Autodesk Inventor part; units mm, degrees
ref_plane "YZ Plane" through (0, 0, 0) normal (1, 0, 0) x (0, 1, 0)
ref_plane "XZ Plane" through (0, 0, 0) normal (0, 1, 0) x (-1, 0, 0)
ref_plane "XY Plane" through (0, 0, 0) normal (0, 0, 1) x (1, 0, 0)
sketch "Esboço1" plane through (0, 0, 0) normal (0, 1, 0) x (-1, 0, 0)
  line L0 (-29, 17) -> (29, 17)
  line L1 (29, 17) -> (29, -17)
  line L2 (29, -17) -> (-29, -17)
  line L3 (-29, -17) -> (-29, 17)
  line L4 (-29, 17) -> (29, -17) construction
  line L5 (29, 17) -> (-29, -17) construction
  point P0 (0, 0)
  point P1 (0.0565, -0.0161)
  dimension "d0" = 58
  dimension "d1" = 34
extrude "Extrusão1" add sketch "Esboço1" along normal blind 3
sketch "Esboço2" plane through (0, 3, 0) normal (0, 1, 0) x (1, 0, 0)
  line L0 (26.5, -14.5) -> (-26.5, -14.5)
  line L1 (-26.5, -14.5) -> (-26.5, 14.5)
  line L2 (-26.5, 14.5) -> (26.5, 14.5)
  line L3 (26.5, 14.5) -> (26.5, -14.5)
  line L4 (26.5, -14.5) -> (-26.5, 14.5) construction
  line L5 (-26.5, -14.5) -> (26.5, 14.5) construction
  line L6 (29, 17) -> (-29, 17)
  line L7 (29, -17) -> (-29, -17)
  line L8 (-29, -17) -> (-29, 17)
  line L9 (-29, 17) -> (29, 17)
  line L10 (29, 17) -> (29, -17)
  line L11 (29, -17) -> (-29, 17) construction
  line L12 (-29, -17) -> (29, 17) construction
  point P0 (0, 0)
  dimension "d4" = 53
  dimension "d5" = 29
extrude "Extrusão2" add sketch "Esboço2" along normal blind 9.5
sketch "Esboço3" plane through (0, 3, 0) normal (0, 1, 0) x (1, 0, 0)
  line L0 (-26.5, 14.5) -> (26.5, 14.5)
  line L1 (-26.5, -14.5) -> (-26.5, 14.5)
  line L2 (26.5, 14.5) -> (26.5, -14.5)
  line L3 (26.5, -14.5) -> (-26.5, -14.5)
  line L4 (-23.5, -14.5) -> (-26.5, -14.5)
  line L5 (-26.5, -14.5) -> (-26.5, -11.5)
  line L6 (-26.5, -11.5) -> (-23.5, -11.5)
  line L7 (-23.5, -11.5) -> (-23.5, -14.5)
  line L8 (-23.5, -14.5) -> (-26.5, -11.5) construction
  line L9 (-26.5, -14.5) -> (-23.5, -11.5) construction
  line L10 (-23.5, 11.5) -> (-26.5, 11.5)
  line L11 (-26.5, 11.5) -> (-26.5, 14.5)
  line L12 (-26.5, 14.5) -> (-23.5, 14.5)
  line L13 (-23.5, 14.5) -> (-23.5, 11.5)
  line L14 (-23.5, 11.5) -> (-26.5, 14.5) construction
  line L15 (-26.5, 11.5) -> (-23.5, 14.5) construction
  line L16 (26.5, -14.5) -> (23.5, -14.5)
  line L17 (23.5, -14.5) -> (23.5, -11.5)
  line L18 (23.5, -11.5) -> (26.5, -11.5)
  line L19 (26.5, -11.5) -> (26.5, -14.5)
  line L20 (26.5, -14.5) -> (23.5, -11.5) construction
  line L21 (23.5, -14.5) -> (26.5, -11.5) construction
  line L22 (26.5, 11.5) -> (23.5, 11.5)
  line L23 (23.5, 11.5) -> (23.5, 14.5)
  line L24 (23.5, 14.5) -> (26.5, 14.5)
  line L25 (26.5, 14.5) -> (26.5, 11.5)
  line L26 (26.5, 11.5) -> (23.5, 14.5) construction
  line L27 (23.5, 11.5) -> (26.5, 14.5) construction
  point P0 (0, 0)
  point P1 (-13.75, -16.75)
  point P2 (-13.75, 16.75)
  point P3 (13.75, 16.75)
  point P4 (13.75, -16.75)
  point P5 (-26.5, -13)
  dimension "d66" = 3
  dimension "d67" = 3
  dimension "d68" = 3
  dimension "d69" = 3
  dimension "d70" = 3
  dimension "d71" = 3
  dimension "d72" = 3
  dimension "d73" = 3
  dimension "d74" = 0
  dimension "d75" = 0
  dimension "d76" = 0
  dimension "d77" = 0
  dimension "d78" = 0
  dimension "d79" = 0
  dimension "d80" = 0
  dimension "d81" = 0
extrude "Extrusão3" add sketch "Esboço3" along normal blind 2 contours L0 L13 L10 L1 | L0 L2 L22 L23 | L6 L7 L3 L1 | L2 L3 L17 L18
chamfer "Chanfro1" distance 2 angle 45 4 edges at (29, 6.25, 17) (-29, 6.25, 17) (-29, 6.25, -17) (29, 6.25, -17)
sketch "Esboço7" plane through (29, 0, 15) normal (1, 0, 0) x (0, 0, -1)
  line L0 (30, 0) -> (0, 0)
  line L1 (0, 0) -> (30, 0)
  line L2 (30, 0) -> (30, 3)
  line L3 (30, 3) -> (0, 3)
  line L4 (0, 3) -> (0, 0)
  line L5 (30, 12.5) -> (30, 0)
  line L6 (0, 0) -> (0, 12.5)
  point P0 (15, 0)
  point P1 (15, 0)
  point P2 (15, 3)
  dimension "d36" = 3
  dimension "d42" = 0
  dimension "d43" = 0
extrude "Extrusão6" add sketch "Esboço7" along normal blind 42.04
sketch "Esboço9" plane through (-29, 0, -15) normal (-1, 0, 0) x (0, 0, 1)
  line L0 (30, 12.5) -> (30, 0)
  line L1 (1.5, 0) -> (30, 0)
  line L2 (30, 0) -> (30, 3)
  line L3 (30, 3) -> (1.5, 3)
  line L4 (1.5, 3) -> (1.5, 0)
  point P0 (15, 0)
  dimension "d59" = 3
extrude "Extrusão8" add sketch "Esboço9" along normal blind 42.04
sketch "Esboço8" plane through (29, 3, 15) normal (0, 1, 0) x (1, 0, 0)
  circle A0 centre (37.5465, 14.25) radius 1.5
  line L0 (0, 0) -> (0, 30)
  line L1 (23.7495, 2) -> (8.7495, 2)
  line L2 (8.7495, 2) -> (8.7495, 28)
  line L3 (8.7495, 28) -> (23.7495, 28)
  line L4 (23.7495, 28) -> (23.7495, 2)
  line L5 (0, 0) -> (42.04, 0)
  line L6 (0, 30) -> (42.04, 30)
  line L7 (-2, 32) -> (-56, 32)
  line L8 (-56, -2) -> (-2, -2)
  circle A1 centre (-95.0465, 14.25) radius 1.5
  line L9 (-81.2495, 2) -> (-66.2495, 2)
  line L10 (-66.2495, 2) -> (-66.2495, 26.5)
  line L11 (-66.2495, 26.5) -> (-81.2495, 26.5)
  line L12 (-81.2495, 26.5) -> (-81.2495, 2)
  point P0 (-29, 15)
  point P1 (23.7495, 15)
  point P2 (-81.2495, 14.25)
  dimension "d44" = 3
  dimension "d47" = 13.797
  dimension "d53" = 2
  dimension "d54" = 2
  dimension "d55" = 15
extrude "Extrusão7" cut sketch "Esboço8" against normal blind 42.04
chamfer "Chanfro2" distance 10 angle 45 4 edges at (71.04, 1.5, -15) (71.04, 1.5, 15) (-71.04, 1.5, -13.5) (-71.04, 1.5, 15)
sketch "Esboço10" plane through (29, 12.5, 15) normal (1, 0, 0) x (0, 0, -1)
  line L0 (0, -9.5) -> (30, -9.5)
  line L1 (30, 0) -> (30, -9.5)
  line L2 (0, 0) -> (30, 0)
  line L3 (0, -9.5) -> (0, 0)
  line L4 (10, -12.5) -> (10, -9.5)
  line L5 (10, -12.5) -> (20, -12.5)
  line L6 (20, -9.5) -> (20, -12.5)
  line L7 (20, -9.5) -> (10, -9.5)
  line L8 (5, -9.5) -> (20, -9.5)
  line L9 (20, -9.5) -> (20, -4.5)
  line L10 (20, -4.5) -> (10, -4.5)
  line L11 (10, -4.5) -> (10, -9.5)
  point P0 (15, -12.5)
  point P1 (20, -9.5)
  point P2 (15, 0)
  point P3 (15, -4.5)
  dimension "d82" = 10
  dimension "d83" = 0
  dimension "d84" = 4.5
  dimension "d85" = 0
  dimension "d86" = 5
extrude "Extrusão9" cut sketch "Esboço10" against normal blind 10 contours L11 L10 L9 L0
chamfer "Chanfro3" distance 3 angle 45 4 edges at (-23.5, 4, 11.5) (-23.5, 4, -11.5) (23.5, 4, -11.5) (23.5, 4, 11.5)
fillet "Arredondamento1" radius 2 8 edges at (-37.2495, 1.5, -11.5) (-37.2495, 1.5, 13) (-52.2495, 1.5, -11.5) (-52.2495, 1.5, 13) (37.7495, 1.5, -13) (37.7495, 1.5, 13) (52.7495, 1.5, -13) (52.7495, 1.5, 13)
fillet "Arredondamento2" radius 2 8 edges at (71.04, 1.5, -5) (71.04, 1.5, 5) (61.04, 1.5, -15) (61.04, 1.5, 15) (-61.04, 1.5, -13.5) (-71.04, 1.5, -3.5) (-71.04, 1.5, 5) (-61.04, 1.5, 15)
properties part number "espbase"
Could you check a few things on this model? Use its own coordinates, in mm. A direction names the side the tool comes from. Give positions to 0.01 mm unless a question says otherwise; leave off trailing zeros. Order: outer loops, then holes, each group sorted by start corner. A loop starts at its lowest first (then second) coordinate and runs counter-clockwise, first axis right, second up. Notation, with made-up numbers: (19, 8) - (31, 8) arc R8 ccw to (31, 13) - close; hole circle Ø4 at (-9, -20). An arc over 180 degrees is marked (long way). Return JSON: item names as keys, results as strings. Group by question number.
Q1. Suppose I cut it at B-B, the plane y = 10.25. Please give me the cut outline in (x, z).
Q2. Thinking about a two-plate mould opening in Z: for faces 1 (the face through (-54, 3, 1)), 2 (the face through (44, 1, -15)), 3 (the face through (28, 6, 5)), which applies, pulls with the +Z half, pulls with the -Z half, needs draft (parallel to the pull), parting line crosses it, or undercut?
Q3. Which directions (+Z, -Z, +X, -X, +Y, -Y) give clear straight access to the entire face, cutting with the end or side of a thin tool? Please do faces 4 (the face through (44, 2, 15)), 5 (the face through (-37.25, 2, 1)), 6 (the face through (29, 9, 0)), 7 (the face through (26.5, 9, 0)).
Q4. Please list where these lines run through material, in increasing order: line 1 along X through (y, z) = (1.2, 0.75); line 2 along Z through (x, y) = (6, 6.25); line 3 along X through (y, z) = (2.75, -6.5). Write a range as [from, to].
Q5. Will these pins go through, and if not, where does the flat tip stop? pin 1 Ø1.5 at (x, y) = (46, 1) entering from +Z; pin 2 Ø2 at (y, z) = (1.5, -11.5) entering from +X; pin 3 Ø1.5 at (x, z) = (-25.5, 12.5) entering from +Y.
Q6. Suppose I cut it at D-D, the plane x = 13. Please give me the cut outline in (y, z).
Q7. Suppose I cut it at A-A, the plane z = 0.75. Please give me the cut outline in (x, y), and give its area (3 significant figures).
Q8. Suppose I cut it at C-C, the plane x = 48.5. Please give me the cut outline in (y, z), and give its area (3 significant figures).
Resolved:
{
 "1": {"outline": "(-29, -15) - (-27, -17) - (27, -17) - (29, -15) - (29, 15) - (27, 17) - (-27, 17) - (-29, 15) - close; hole (-26.5, -14.5) - (26.5, -14.5) - (26.5, 14.5) - (-26.5, 14.5) - close"},
 "2": {"face 1": "needs draft", "face 2": "pulls with the -Z half", "face 3": "undercut"},
 "3": {"face 4": "+Z, +X, +Y, -Y", "face 5": "+Y, -Y", "face 6": "+Z, -Z, +X, +Y", "face 7": "+Y"},
 "4": {"line 1": "x = [-71.04, -67.55], [-64.55, -52.25], [-37.25, 37.75], [52.75, 65.05], [68.05, 71.04]", "line 2": "z = [-17, -14.5], [14.5, 17]", "line 3": "x = [-68.04, -52.25], [-37.25, 37.75], [52.75, 69.54]"},
 "5": {"pin 1": "stops at z = 15", "pin 2": "stops at x = 65.54", "pin 3": "stops at y = 5"},
 "6": {"outline": "(0, -17) - (12.5, -17) - (12.5, -14.5) - (3, -14.5) - (3, 14.5) - (12.5, 14.5) - (12.5, 17) - (0, 17) - close"},
 "7": {"outline": "(-71.04, 0) - (-67.55, 0) - (-67.55, 3) - (-71.04, 3) - close; (-64.55, 0) - (-52.25, 0) - (-52.25, 3) - (-64.55, 3) - close; (-37.25, 0) - (37.75, 0) - (37.75, 3) - (-26.5, 3) - (-26.5, 12.5) - (-29, 12.5) - (-29, 3) - (-37.25, 3) - close; (26.5, 8) - (29, 8) - (29, 12.5) - (26.5, 12.5) - close; (52.75, 0) - (65.05, 0) - (65.05, 3) - (52.75, 3) - close; (68.05, 0) - (71.04, 0) - (71.04, 3) - (68.05, 3) - close", "area": "353 mm2"},
 "8": {"outline": "(0, -15) - (3, -15) - (3, -13) - (0, -13) - close; (0, 13) - (3, 13) - (3, 15) - (0, 15) - close", "area": "12.0 mm2"}
}
